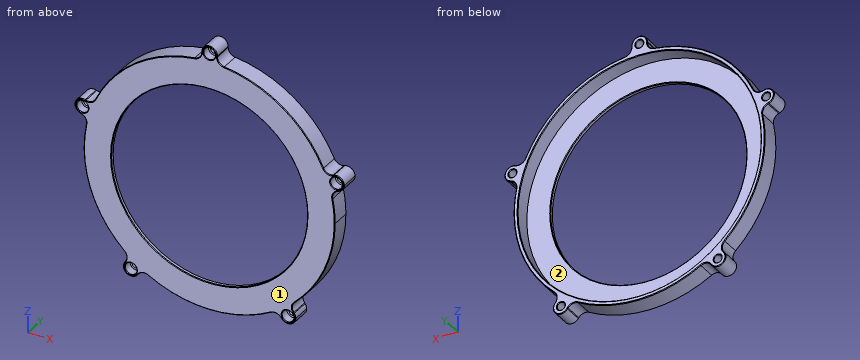
```python
from build123d import *

# Parameters (mm, degrees)
F0_R     = 3.175
F0_R_2   = 98.425
F1_DEPTH = 15.875
F0_R_3   = 79.375
F2_DEPTH = 3.175
F3_R     = 6.35
F4_R     = 4.7625
F4_R_2   = 3.175
F5_DEPTH = 7.112
F6_SIZE  = 0.508


with BuildPart() as f1:
    # F0 (on Front) → F1 (new body)
    with BuildSketch(Plane.XZ):
        with BuildLine():
            ThreePointArc((94.476174201, 37.3739549465), (95.5984942164, 34.401859013), (96.6273421242, 31.3961264172))
            ThreePointArc((96.6273421242, 31.3961264172), (97.008659455, 36.2412241172), (100.7042930198, 39.3975934212))
            Line((100.7042930198, 39.3975934212), (94.476174201, 37.3739549465))
        make_face()
        with BuildLine():
            ThreePointArc((96.6273421242, 31.3961264172), (97.5617118991, 28.3596962488), (98.4006900295, 25.2955371896))
            Line((98.4006900295, 25.2955371896), (104.6288088483, 27.3191756643))
            ThreePointArc((104.6288088483, 27.3191756643), (99.7837113597, 27.7004930638), (96.6273421242, 31.3961264172))
        make_face()
        with BuildLine():
            ThreePointArc((100.7042930198, 39.3975934212), (97.008659455, 36.2412241172), (96.6273421242, 31.3961264172))
            ThreePointArc((96.6273421242, 31.3961264172), (99.7837113597, 27.7004930638), (104.6288088483, 27.3191756643))
            ThreePointArc((104.6288088483, 27.3191756643), (107.8038088483, 29.6259481907), (109.0165509341, 33.3583845428))
            ThreePointArc((109.0165509341, 33.3583845428), (106.3989872861, 38.4956424571), (100.7042930198, 39.3975934212))
        make_face()
        with Locations((102.6665509341, 33.3583845428)):
            Circle(F0_R, mode=Mode.SUBTRACT)
        with BuildLine():
            Line((68.5886758993, -83.6009481907), (64.7394867833, -78.302993883))
            ThreePointArc((64.7394867833, -78.302993883), (62.2596715502, -80.2888117888), (59.7189814811, -82.1961267388))
            ThreePointArc((59.7189814811, -82.1961267388), (64.4447767453, -81.0615635653), (68.5886758993, -83.6009481907))
        make_face()
        with BuildLine():
            ThreePointArc((68.5886758993, -83.6009481907), (64.4447767453, -81.0615635653), (59.7189814811, -82.1961267388))
            ThreePointArc((59.7189814811, -82.1961267388), (57.1795970075, -86.3400257824), (58.3141600707, -91.0658208948))
            ThreePointArc((58.3141600707, -91.0658208948), (65.4136758993, -93.3725934212), (69.801417985, -87.3333845428))
            ThreePointArc((69.801417985, -87.3333845428), (69.4906268634, -85.3711266285), (68.5886758993, -83.6009481907))
        make_face()
        with Locations((63.451417985, -87.3333845428)):
            Circle(F0_R, mode=Mode.SUBTRACT)
        with BuildLine():
            ThreePointArc((58.3141600707, -91.0658208948), (57.1795970075, -86.3400257824), (59.7189814811, -82.1961267388))
            ThreePointArc((59.7189814811, -82.1961267388), (57.119900909, -84.0230737366), (54.4649709547, -85.7678665871))
            Line((54.4649709547, -85.7678665871), (58.3141600707, -91.0658208948))
        make_face()
        with BuildLine():
            Line((-58.3141600707, -91.0658208948), (-54.4649709547, -85.7678665871))
            ThreePointArc((-54.4649709547, -85.7678665871), (-57.1199011195, -84.0230735935), (-59.7189818929, -82.1961264396))
            ThreePointArc((-59.7189818929, -82.1961264396), (-57.7935266293, -84.4505447262), (-57.101417985, -87.3333845428))
            ThreePointArc((-57.101417985, -87.3333845428), (-57.4122091065, -89.2956424571), (-58.3141600707, -91.0658208948))
        make_face()
        with BuildLine():
            ThreePointArc((-68.5886758993, -83.6009481907), (-64.4447769967, -81.0615636051), (-59.7189818929, -82.1961264396))
            ThreePointArc((-59.7189818929, -82.1961264396), (-62.2596717513, -80.2888116329), (-64.7394867833, -78.302993883))
            Line((-64.7394867833, -78.302993883), (-68.5886758993, -83.6009481907))
        make_face()
        with BuildLine():
            ThreePointArc((-57.101417985, -87.3333845428), (-57.7935266293, -84.4505447262), (-59.7189818929, -82.1961264396))
            ThreePointArc((-59.7189818929, -82.1961264396), (-64.4447769967, -81.0615636051), (-68.5886758993, -83.6009481907))
            ThreePointArc((-68.5886758993, -83.6009481907), (-67.183854337, -92.4706424571), (-58.3141600707, -91.0658208948))
            ThreePointArc((-58.3141600707, -91.0658208948), (-57.4122091065, -89.2956424571), (-57.101417985, -87.3333845428))
        make_face()
        with Locations((-63.451417985, -87.3333845428)):
            Circle(F0_R, mode=Mode.SUBTRACT)
        with BuildLine():
            ThreePointArc((-104.6288088483, 27.3191756643), (-99.7837113781, 27.7004930543), (-96.627342137, 31.3961263778))
            ThreePointArc((-96.627342137, 31.3961263778), (-96.3947299919, 32.3650255596), (-96.3165509341, 33.3583845428))
            ThreePointArc((-96.3165509341, 33.3583845428), (-97.5292930198, 37.0908208948), (-100.7042930198, 39.3975934212))
            ThreePointArc((-100.7042930198, 39.3975934212), (-108.7057598125, 35.3206424571), (-104.6288088483, 27.3191756643))
        make_face()
        with Locations((-102.6665509341, 33.3583845428)):
            Circle(F0_R, mode=Mode.SUBTRACT)
        with BuildLine():
            ThreePointArc((-96.627342137, 31.3961263778), (-95.5984942234, 34.4018589935), (-94.476174201, 37.3739549465))
            Line((-94.476174201, 37.3739549465), (-100.7042930198, 39.3975934212))
            ThreePointArc((-100.7042930198, 39.3975934212), (-97.5292930198, 37.0908208948), (-96.3165509341, 33.3583845428))
            ThreePointArc((-96.3165509341, 33.3583845428), (-96.3947299919, 32.3650255596), (-96.627342137, 31.3961263778))
        make_face()
        with BuildLine():
            Line((-104.6288088483, 27.3191756643), (-98.4006900295, 25.2955371896))
            ThreePointArc((-98.4006900295, 25.2955371896), (-97.5617119048, 28.3596962289), (-96.627342137, 31.3961263778))
            ThreePointArc((-96.627342137, 31.3961263778), (-99.7837113781, 27.7004930543), (-104.6288088483, 27.3191756643))
        make_face()
        with BuildLine():
            ThreePointArc((-6.35, 107.95), (-4.490128111, 103.4598719899), (-1.426e-07, 101.6))
            ThreePointArc((-1.426e-07, 101.6), (4.4901280101, 103.459871889), (6.35, 107.95))
            ThreePointArc((6.35, 107.95), (0, 114.3), (-6.35, 107.95))
        make_face()
        with Locations((0, 107.95)):
            Circle(F0_R, mode=Mode.SUBTRACT)
        with BuildLine():
            ThreePointArc((-1.426e-07, 101.6), (3.1765528772, 101.5503299444), (6.35, 101.401368334))
            Line((6.35, 101.401368334), (6.35, 107.95))
            ThreePointArc((6.35, 107.95), (4.4901280101, 103.459871889), (-1.426e-07, 101.6))
        make_face()
        with BuildLine():
            ThreePointArc((-6.35, 101.401368334), (-3.1765530198, 101.5503299399), (-1.426e-07, 101.6))
            ThreePointArc((-1.426e-07, 101.6), (-4.490128111, 103.4598719899), (-6.35, 107.95))
            Line((-6.35, 107.95), (-6.35, 101.401368334))
        make_face()
        with BuildLine():
            ThreePointArc((64.7394867833, -78.302993883), (91.9241313725, -43.2725556376), (101.6, 0))
            ThreePointArc((101.6, 0), (100.7969992287, 12.7485272286), (98.4006900295, 25.2955371896))
            ThreePointArc((98.4006900295, 25.2955371896), (97.5617118991, 28.3596962488), (96.6273421242, 31.3961264172))
            ThreePointArc((96.6273421242, 31.3961264172), (95.5984942164, 34.401859013), (94.476174201, 37.3739549465))
            ThreePointArc((94.476174201, 37.3739549465), (59.7189816329, 82.1961266285), (6.35, 101.401368334))
            ThreePointArc((6.35, 101.401368334), (3.1765528772, 101.5503299444), (-1.426e-07, 101.6))
            ThreePointArc((-1.426e-07, 101.6), (-3.1765530198, 101.5503299399), (-6.35, 101.401368334))
            ThreePointArc((-6.35, 101.401368334), (-59.7189816329, 82.1961266285), (-94.476174201, 37.3739549465))
            ThreePointArc((-94.476174201, 37.3739549465), (-95.5984942234, 34.4018589935), (-96.627342137, 31.3961263778))
            ThreePointArc((-96.627342137, 31.3961263778), (-97.5617119048, 28.3596962289), (-98.4006900295, 25.2955371896))
            ThreePointArc((-98.4006900295, 25.2955371896), (-96.6273420556, -31.3961266285), (-64.7394867833, -78.302993883))
            ThreePointArc((-64.7394867833, -78.302993883), (-62.2596717513, -80.2888116329), (-59.7189818929, -82.1961264396))
            ThreePointArc((-59.7189818929, -82.1961264396), (-57.1199011195, -84.0230735935), (-54.4649709547, -85.7678665871))
            ThreePointArc((-54.4649709547, -85.7678665871), (0, -101.6), (54.4649709547, -85.7678665871))
            ThreePointArc((54.4649709547, -85.7678665871), (57.119900909, -84.0230737366), (59.7189814811, -82.1961267388))
            ThreePointArc((59.7189814811, -82.1961267388), (62.2596715502, -80.2888117888), (64.7394867833, -78.302993883))
        make_face()
        Circle(F0_R_2, mode=Mode.SUBTRACT)
    extrude(amount=-F1_DEPTH)

    # F0 (on Front) → F2 (join)
    with BuildSketch(Plane.XZ):
        Circle(F0_R_2)
        Circle(F0_R_3, mode=Mode.SUBTRACT)
    extrude(amount=-F2_DEPTH)

    # F3
    f3_edges = [f1.edges().sort_by_distance(p)[0] for p in [
        (-98.40069, 7.9375, 25.295537),
        (-64.739487, 7.9375, -78.302994),
        (-54.464971, 7.9375, -85.767867),
        (54.464971, 7.9375, -85.767867),
        (64.739487, 7.9375, -78.302994),
        (94.476174, 7.9375, 37.373955),
        (6.35, 7.9375, 101.401368),
        (-6.35, 7.9375, 101.401368),
        (-94.476174, 7.9375, 37.373955),
        (98.40069, 7.9375, 25.295537),
    ]]
    fillet(f3_edges, radius=F3_R)

    # F4 (on face) → F5 (cut)
    with BuildSketch(Plane.XZ):
        with Locations((-63.451417985, -87.3333845428)):
            Circle(F4_R)
        with Locations((-63.451417985, -87.3333845428)):
            Circle(F4_R_2, mode=Mode.SUBTRACT)
        with Locations((-102.6665509341, 33.3583845428)):
            Circle(F4_R)
        with Locations((-102.6665509341, 33.3583845428)):
            Circle(F4_R_2, mode=Mode.SUBTRACT)
        with Locations((0, 107.95)):
            Circle(F4_R)
        with Locations((0, 107.95)):
            Circle(F4_R_2, mode=Mode.SUBTRACT)
        with Locations((102.6665509341, 33.3583845428)):
            Circle(F4_R)
        with Locations((102.6665509341, 33.3583845428)):
            Circle(F4_R_2, mode=Mode.SUBTRACT)
        with Locations((63.451417985, -87.3333845428)):
            Circle(F4_R)
        with Locations((63.451417985, -87.3333845428)):
            Circle(F4_R_2, mode=Mode.SUBTRACT)
    extrude(amount=-F5_DEPTH, mode=Mode.SUBTRACT)

    # F6
    f6_edges = [f1.edges().sort_by_distance(p)[0] for p in [
        (-59.718982, 0, 82.196127),
        (-96.627342, 15.875, -31.396127),
        (-79.375, 3.175, 0),
        (-79.375, 0, 0),
        (-107.429051, 0, 33.358385),
        (-4.7625, 0, 107.95),
        (-68.213918, 0, -87.333385),
        (97.904051, 0, 33.358385),
        (58.688918, 0, -87.333385),
        (-98.425, 15.875, 0),
        (-3.175, 15.875, 107.95),
        (-105.841551, 15.875, 33.358385),
        (-66.626418, 15.875, -87.333385),
        (60.276418, 15.875, -87.333385),
        (99.491551, 15.875, 33.358385),
    ]]
    chamfer(f6_edges, length=F6_SIZE)


solid = f1.part
```
Can you work these out from the model? Positions are in its coordinate system, mm. Face numbers are marked on the shaded views. Give positions to 0.01 mm unless a question says otherwise; leave off trailing zeros. One line per item, written item: value.
Q1. Please list where these lines run through material, in increasing order: line 1 (Z direction, x = 0, y = 1) (1 decimal); line 2 (X direction, y = 13, z = 107.95) (3 decimals); line 3 (X direction, y = 6, z = -91). Write a range as [from, to].
Results found:
line 1: z = [-101.6, -79.4], [79.4, 103.2], [112.7, 114.3]
line 2: x = [-6.35, -3.175], [3.175, 6.35]
line 3: x = [-68.64, -66.49], [-60.41, -58.27], [-45.18, -37.5], [37.5, 45.18], [58.27, 60.41], [66.49, 68.64]
Q2. We'd pull the mould along X, two halves only. Please class the marked faces 1 and 2: +X half, -X half, draft (parallel to the pull), parting line (faces both ways), or undercut.
Results found:
face 1: draft
face 2: undercut
Q3. For P1, Ø5, axis at x = 0.5, z = 105.5, coming from the -Y side; P2, Ø5, axis at x = -63.45, z = -87.33, coming from the -Y side; P3, Ø7.5, axis at x = 102.67, z = 33.36, coming from the -Y side; P4, Ø8, axis at x = -49.5, y = 13.5, coming from the +Z side, each with a flat end and sliding along its axis, tell me the tip position at first contact or that it passes through.
Results found:
P1: stops at y = 0.27
P2: passes through
P3: stops at y = 7.11
P4: stops at z = 90.84
Q4. Imagine slicing it at A-A on x = 0. Give the number of separate pieces and of enclosed holes in the cut face, and give its area (3 significant figures).
Results found:
separate pieces: 3
enclosed holes: 0
area: 298 mm^2
